Here's how the part is built. I have some questions about the finished solid (model axes, mm). A direction names the side the tool comes from. Coordinates: 2 decimals unless noted, no trailing zeros. Loops run counter-clockwise (first coordinate to the right, second up) from the corner with the lowest first, then second, coordinate; pieces in that order, holes last. Notation, with made-up numbers: (49, 5) - (102, 5) arc R14 cw to (102, 11) - close; hole circle Ø5 at (-29, -4). An arc over 180 degrees is marked (long way). Use a Markdown table: item, result.
Autodesk Inventor part; units mm, degrees
ref_plane "YZ Plane" through (0, 0, 0) normal (1, 0, 0) x (0, 1, 0)
ref_plane "XZ Plane" through (0, 0, 0) normal (0, 1, 0) x (-1, 0, 0)
ref_plane "XY Plane" through (0, 0, 0) normal (0, 0, 1) x (1, 0, 0)
sketch "Sketch1" plane through (0, 0, 0) normal (0, 1, 0) x (-1, 0, 0)
  line L0 (43.7447, 29.8192) -> (-47.6553, 29.8192)
  line L1 (-47.6553, 29.8192) -> (-47.6553, -33.0808)
  line L2 (-47.6553, -33.0808) -> (43.7447, -33.0808)
  line L3 (43.7447, -33.0808) -> (43.7447, 29.8192)
  line L4 (53.7447, 39.8192) -> (-57.6553, 39.8192)
  line L5 (-57.6553, 39.8192) -> (-57.6553, -43.0808)
  line L6 (-57.6553, -43.0808) -> (53.7447, -43.0808)
  line L7 (53.7447, -43.0808) -> (53.7447, 39.8192)
  line L8 (43.7447, 29.8192) -> (43.7447, 39.8192)
  line L9 (-47.6553, 29.8192) -> (-47.6553, 39.8192)
  line L10 (43.7447, -25.8728) -> (15.7447, -25.8728)
  arc A0 (22.3207, -16.6423) -> (18.5901, -33.0808) centre (33.3129, -27.7795) ccw
  arc A1 (23.9512, -1.3415) -> (22.3207, -16.6423) centre (31.8383, -9.9192) ccw
  arc A2 (29.8207, 14.6173) -> (23.9512, -1.3415) centre (35.1226, 3.6085) ccw
  arc A3 (43.7447, 39.8192) -> (29.8207, 14.6173) centre (50.0285, 19.8999) ccw
  point P0 (0, 0)
  point P1 (42.359, 39.8192)
  point P2 (31.6472, 29.8192)
  dimension "d0" = 91.4
  dimension "d1" = 62.9
  dimension "d2" = 10
  dimension "d17" = 28
extrude "Extrusion1" add sketch "Sketch1" along normal blind 5 contours L3 L10 A0 A1 A2 A3 L0 | L8 L4 L7 L6 L5 L9 L1 L2 L3 | L0 A3 L8 | L3 L2 A0 L10
fillet "Fillet1" radius 10 4 edges at (57.6553, 2.5, 39.8192) (-53.7447, 2.5, 39.8192) (57.6553, 2.5, -43.0808) (-53.7447, 2.5, -43.0808)
sketch "Sketch2" plane through (0, 0, 0) normal (0, -1, 0) x (1, 0, 0)
  arc A0 (-53.7447, -33.0808) -> (-43.7447, -43.0808) centre (-43.7447, -33.0808) ccw
  line L0 (47.6553, -43.0808) -> (-43.7447, -43.0808)
  arc A1 (47.6553, -43.0808) -> (57.6553, -33.0808) centre (47.6553, -33.0808) ccw
  line L1 (57.6553, 29.8192) -> (57.6553, -33.0808)
  arc A2 (57.6553, 29.8192) -> (47.6553, 39.8192) centre (47.6553, 29.8192) ccw
  arc A3 (-43.7447, 39.8192) -> (-53.7447, 29.8192) centre (-43.7447, 29.8192) ccw
  line L2 (-53.7447, -33.0808) -> (-53.7447, 29.8192)
  line L3 (47.6553, -33.0808) -> (47.6553, 39.8192)
  line L4 (54.7263, 36.8902) -> (51.1908, 33.3547)
  line L5 (54.7263, -40.1519) -> (51.1908, -36.6164)
  line L6 (-50.8158, 36.8902) -> (-47.2803, 33.3547)
  line L7 (-50.8158, -40.1519) -> (-47.2803, -36.6164)
  circle A4 centre (-47.2803, -36.6164) radius 1.45
  circle A5 centre (-47.2803, 33.3547) radius 1.45
  circle A6 centre (51.1908, 33.3547) radius 1.45
  circle A7 centre (51.1908, -36.6164) radius 1.45
  arc A8 (-29.8207, 14.6173) -> (-43.7447, 39.8192) centre (-50.0285, 19.8999) ccw
  line L8 (-18.5901, -33.0808) -> (47.6553, -33.0808)
  arc A9 (-18.5901, -33.0808) -> (-22.3207, -16.6423) centre (-33.3129, -27.7795) ccw
  arc A10 (-22.3207, -16.6423) -> (-23.9512, -1.3415) centre (-31.8383, -9.9192) ccw
  arc A11 (-23.9512, -1.3415) -> (-29.8207, 14.6173) centre (-35.1226, 3.6085) ccw
  point P0 (0, 0)
  dimension "d6" = 5
  dimension "d7" = 5
  dimension "d8" = 5
  dimension "d9" = 5
  dimension "d10" = 2.9
  dimension "d11" = 2.9
  dimension "d12" = 2.9
  dimension "d13" = 2.9
extrude "Extrusion2" cut sketch "Sketch2" against normal blind 3 contours A4 | A7 | A6 | A5
fillet "Fillet2" radius 3 4 edges at (-43.7447, 2.5, 39.8192) (-43.7452, 2.5, 39.8192) (47.6558, 2.5, 39.8192) (47.6553, 2.5, 39.8192)
sketch "Sketch3" plane through (0, 5, 0) normal (0, 1, 0) x (1, 0, 0)
  arc A0 (-22.3207, 16.6423) -> (-18.5901, 33.0808) centre (-33.3129, 27.7795) ccw
  circle A1 centre (-33.3129, 27.7795) radius 15.6482
  line L0 (-18.5901, 33.0808) -> (47.6553, 33.0808)
  line L1 (47.6553, 33.0808) -> (-20.0549, 33.0808)
  line L2 (-20.0549, 33.0808) -> (-20.0549, 37.0808)
  line L3 (-20.0549, 37.0808) -> (47.6553, 37.0808)
  line L4 (47.6553, 37.0808) -> (47.6553, 33.0808)
  point P0 (0, 0)
  point P1 (-20.0549, 36.0916)
  dimension "d18" = 4
extrude "Extrusion3" cut sketch "Sketch3" against normal blind 10 contours L2 L3 L4 L0 A1
fillet "Fillet3" radius 2 6 edges at (-20.0549, 2.5, -37.0808) (-20.0549, 2.5, -36.0916) (47.6553, 2.5, -37.0808) (-29.8207, 2.5, 14.6173) (-23.9512, 2.5, -1.3415) (-22.3207, 2.5, -16.6423)
properties part number "Top"
Q1. Please list where these lines run through material, in increasing order: L1, parallel to X at y = 2.2, z = 4; L2, parallel to Z at x = -48, y = 1.8; L3, parallel to X at y = 1.5, z = -10. Write a range as from..to.
Check values:
| item | result |
|---|---|
| L1 | -53.74..-22.91, 47.66..57.66 |
| L2 | -42.13..-37.88, -35.36..32.1, 34.61..38.87 |
| L3 | -53.74..-20.19, 47.66..57.66 |
Q2. Will these pins go through, and if not, where does the flat tip stop? P1, Ø2.5, axis at x = -47.28, z = 33.35, coming from the -Y side; P2, Ø8, axis at x = -28.5, z = 29.5, coming from the -Y side; P3, Ø1.5, axis at x = 22, y = 2.5, coming from the +Z side.
Check values:
| item | result |
|---|---|
| P1 | y = 3 |
| P2 | y = 0 |
| P3 | z = -37.08 |
Q3. I want a section at C-C, the plane x = 10. Write out the boundary of the cut face in (y, z), then the cut area to 3 significant figures.
Check values:
| item | result |
|---|---|
| outline | (0, -43.08) - (5, -43.08) - (5, -37.08) - (0, -37.08) - close |
| area | 30.0 mm^2 |
Q4. I want a section at D-D, the plane y = 1.95. Give the number of separate pieces and of enclosed holes in the cut face, then the cut area to 3 significant figures.
Check values:
| item | result |
|---|---|
| separate pieces | 1 |
| enclosed holes | 4 |
| area | 3,550 mm^2 |
Q5. Which directions (+Z, -Z, +X, -X, +Y, -Y) give clear straight access to the entire face, cutting with the end or side of a thin tool? Please do faces 4 (the face through (-50.738, 2.535, -40.229)), 5 (the face through (-20.25, 2.46, -8.68)), 6 (the face through (14, 3, -37.081)), 7 (the face through (-47, 3, 33)), 8 (the face through (3, 2, -43.081)).
Check values:
| item | result |
|---|---|
| face 4 | -Z, -X, +Y, -Y |
| face 5 | +Y, -Y |
| face 6 | +Z, +Y, -Y |
| face 7 | -Y |
| face 8 | -Z, +X, -X, +Y, -Y |
Q6. If we mould it in two halves opening along X, with no side actions, what happens to faces 1 (the face through (47.655, 2, 1)), 2 (the face through (-51.106, 2.535, 36.587)), 3 (the face through (54.804, 2.535, -40.074))? For each: pulls with the +X half, pulls with the -X half, needs draft (parallel to the pull), parting line crosses it, or undercut.
Check values:
| item | result |
|---|---|
| face 1 | undercut |
| face 2 | pulls with the -X half |
| face 3 | pulls with the +X half |
Q7. I want a section at A-A, the plane z = -14. Write out the boundary of the cut face in (x, y).
Check values:
| item | result |
|---|---|
| outline | (-53.74, 0) - (-20.92, 0) - (-20.92, 5) - (-53.74, 5) - close; (47.66, 0) - (57.66, 0) - (57.66, 5) - (47.66, 5) - close |
Q8. I want a section at B-B, the plane z = 7. Write out the boundary of the cut face in (x, y), then the cut area to 3 significant figures.
Check values:
| item | result |
|---|---|
| outline | (-53.74, 0) - (-23.38, 0) - (-23.38, 5) - (-53.74, 5) - close; (47.66, 0) - (57.66, 0) - (57.66, 5) - (47.66, 5) - close |
| area | 202 mm^2 |
